Could you check a few things on this model? Use its own coordinates, in mm. Face numbers are marked on the shaded views. A direction names the side the tool comes from. Give positions to 0.01 mm unless a question says otherwise; leave off trailing zeros. Order: outer loops, then holes, each group sorted by start corner. A loop starts at its lowest first (then second) coordinate and runs counter-clockwise, first axis right, second up. Notation, with made-up numbers: M 6,81.5 L 13,81.5 A24 cw 13,101.5 Z; hole C 8.5,74 d11. An arc over 180 degrees is marked long. Use a Markdown table: item, result. Add a question column.
Item 1: Suppose I cut it at B-B on x = 458. Write out the boundary of the cut face in (y, z), plus the area to 3 significant figures.
Item 2: For the marked faces 1, 2, 3 and 4, which set-ups out of +Z, -Z, +X, -X, +Y, -Y let a thin tool reach every point of the face, with its end or its side?
Item 3: I'm going to push flat-ended pins straight in: pin 1 Ø6 at (x, y) = (474, -374) entering from +Z; pin 2 Ø21 at (y, z) = (-313, -68.5) entering from -X; pin 3 Ø21 at (x, y) = (77, -261.5) entering from -Z. Where does each tip first touch, or does it pass through?
Item 4: Suppose I cut it at D-D on z = -74.5. Write out the boundary of the cut face in (x, y), plus the area to 3 significant figures.
Item 5: Suppose I cut it at C-C on y = -25. Write out the boundary of the cut face in (x, z), plus the area to 3 significant figures.
Item 6: If we mould it in two halves opening along Z, with no side actions, what happens to the marked faces 5, 6 and 7? For each: released by +Z, released by -Z, zero draft, split by the parting line, or undercut.
Item 7: If I drill on L1, parallel to X at y = -126, z = -189; L2, parallel to Z at x = 128.5, y = -36; L3, parallel to X at y = -248.5, z = -99.5, over which ranges is the centre line in solid material (lowest first)? Write a range as from..to.
Item 8: Suppose I cut it at A-A on y = -304. Write out the boundary of the cut face in (x, z), plus the area to 3 significant figures.
from build123d import *

# Parameters (mm, degrees)
SKETCH1_W           = 540
SKETCH1_H           = 380
BOSS_EXTRUDE1_DEPTH = 140
SKETCH3_W           = 510
SKETCH3_H           = 350
CUT_EXTRUDE1_DEPTH  = 10
SKETCH2_W           = 225
SKETCH2_H           = 320
CUT_EXTRUDE2_DEPTH  = 40
CUT_EXTRUDE3_DEPTH  = 80
FILLET1_R           = 35
SKETCH6_W           = 70
SKETCH6_H           = 70
BOSS_EXTRUDE2_DEPTH = 280


with BuildPart() as part:
    # Sketch1 → Boss-Extrude1 (new body)
    with BuildSketch(Plane(origin=(0, 0, 0), x_dir=(1, 0, 0), z_dir=(0, 1, 0))):
        with Locations((270, 190)):
            Rectangle(SKETCH1_W, SKETCH1_H)
    extrude(amount=-BOSS_EXTRUDE1_DEPTH)

    # Sketch3 → Cut-Extrude1 (cut)
    with BuildSketch(Plane(origin=(0, 0, 0), x_dir=(1, 0, 0), z_dir=(0, 1, 0))):
        with Locations((270, 190)):
            Rectangle(SKETCH3_W, SKETCH3_H)
    extrude(amount=-CUT_EXTRUDE1_DEPTH, mode=Mode.SUBTRACT)

    # Sketch2 → Cut-Extrude2 (cut)
    with BuildSketch(Plane(origin=(0, -10, 0), x_dir=(1, 0, 0), z_dir=(0, 1, 0))):
        with Locations((142.5, 190)):
            Rectangle(SKETCH2_W, SKETCH2_H)
        with Locations((397.5, 190)):
            Rectangle(SKETCH2_W, SKETCH2_H)
    extrude(amount=-CUT_EXTRUDE2_DEPTH, mode=Mode.SUBTRACT)

    # Sketch5 → Cut-Extrude3 (cut)
    with BuildSketch(Plane(origin=(0, -50, 0), x_dir=(1, 0, 0), z_dir=(0, 1, 0))):
        Polygon((30, 290), (90, 350), (255, 350), (255, 30), (90, 30), (30, 90), align=None)
        Polygon((510, 90), (450, 30), (285, 30), (285, 350), (450, 350), (510, 290), align=None)
    extrude(amount=-CUT_EXTRUDE3_DEPTH, mode=Mode.SUBTRACT)

    # Fillet1
    fillet1_edges = [part.edges().sort_by_distance(p)[0] for p in [
        (15, -5, -15),
        (15, -5, -365),
        (525, -5, -365),
        (525, -5, -15),
        (30, -30, -30),
        (30, -30, -350),
        (255, -70, -350),
        (255, -70, -30),
        (510, -30, -350),
        (510, -30, -30),
        (285, -70, -30),
        (285, -70, -350),
        (0, -70, -380),
        (540, -70, -380),
        (540, -70, 0),
        (0, -70, 0),
    ]]
    fillet(fillet1_edges, radius=FILLET1_R)

    # Sketch6 → Boss-Extrude2 (add)
    with BuildSketch(Plane.XZ.offset(140)):
        with Locations((65, -65)):
            Rectangle(SKETCH6_W, SKETCH6_H)
        with Locations((475, -65)):
            Rectangle(SKETCH6_W, SKETCH6_H)
        with Locations((475, -315)):
            Rectangle(SKETCH6_W, SKETCH6_H)
        with Locations((65, -315)):
            Rectangle(SKETCH6_W, SKETCH6_H)
    extrude(amount=BOSS_EXTRUDE2_DEPTH)


solid = part.part
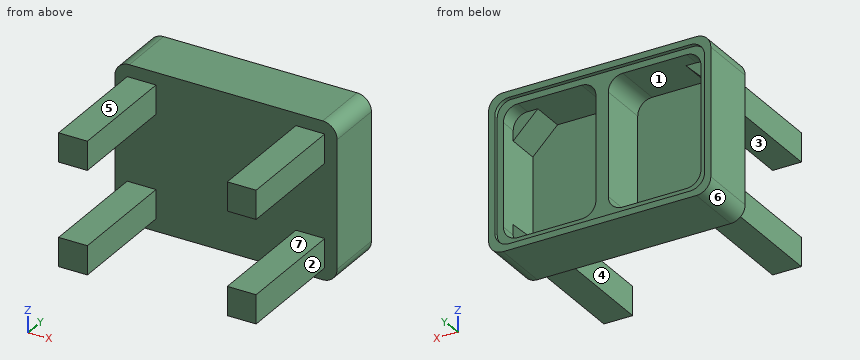
Findings below:
| question | item | result |
|---|---|---|
| 1 | outline | M -420,-350 L -140,-350 L -140,-380 L 0,-380 L 0,-365 L -10,-365 L -10,-350 L -50,-350 L -50,-342 L -130,-342 L -130,-38 L -50,-38 L -50,-30 L -10,-30 L -10,-15 L 0,-15 L 0,0 L -140,0 L -140,-30 L -420,-30 L -420,-100 L -140,-100 L -140,-280 L -420,-280 Z |
| 1 | area | 51,800 mm^2 |
| 2 | face 1 | +Y |
| 2 | face 2 | +Z, -Z, +X, -Y |
| 2 | face 3 | +X, -X, -Y |
| 2 | face 4 | +Z, -Z, -Y |
| 3 | pin 1 | stops at z = -30 |
| 3 | pin 2 | stops at x = 30 |
| 3 | pin 3 | stops at z = -350 |
| 4 | outline | M 0,-140 L 30,-140 L 30,-420 L 100,-420 L 100,-140 L 440,-140 L 440,-420 L 510,-420 L 510,-140 L 540,-140 L 540,0 L 525,0 L 525,-10 L 510,-10 L 510,-50 L 494.5,-50 L 494.5,-130 L 285,-130 L 285,-10 L 255,-10 L 255,-130 L 45.5,-130 L 45.5,-50 L 30,-50 L 30,-10 L 15,-10 L 15,0 L 0,0 Z |
| 4 | area | 58,200 mm^2 |
| 5 | outline | M 0,-345 A35 ccw 35,-380 L 505,-380 A35 ccw 540,-345 L 540,-35 A35 ccw 505,0 L 35,0 A35 ccw 0,-35 Z; hole M 30,-315 A35 ccw 65,-350 L 220,-350 A35 ccw 255,-315 L 255,-65 A35 ccw 220,-30 L 65,-30 A35 ccw 30,-65 Z; hole M 285,-315 A35 ccw 320,-350 L 475,-350 A35 ccw 510,-315 L 510,-65 A35 ccw 475,-30 L 320,-30 A35 ccw 285,-65 Z |
| 5 | area | 62,300 mm^2 |
| 6 | face 5 | released by +Z |
| 6 | face 6 | released by -Z |
| 6 | face 7 | undercut |
| 7 | L1 | x = 0..30, 255..285, 510..540 |
| 7 | L2 | z = -380..-350, -30..0 |
| 7 | L3 | x = 30..100, 440..510 |
| 8 | outline | M 30,-350 L 100,-350 L 100,-280 L 30,-280 Z; M 30,-100 L 100,-100 L 100,-30 L 30,-30 Z; M 440,-350 L 510,-350 L 510,-280 L 440,-280 Z; M 440,-100 L 510,-100 L 510,-30 L 440,-30 Z |
| 8 | area | 19,600 mm^2 |
